Design review of the part built by this model. Coordinates are the model's own, in mm. A direction names the side the tool comes from. Coordinates: 2 decimals unless noted, no trailing zeros. Loops run counter-clockwise (first coordinate to the right, second up) from the corner with the lowest first, then second, coordinate; pieces in that order, holes last.
Q1. Add section C-C on y = -44. Give the boundary of the cut face in (x, z), and give its area (3 significant figures).
Q2. Draft analysis for pull direction Z (two halves, no side actions). For faces 1 (the face through (-0.54, -82.68, -2.44)), 2 (the face through (0, -70, 0)), 3 (the face through (5.15, -53.72, -0.05)), 4 (the face through (-4.76, -46.84, -3.65)), state which applies: released by +Z, released by -Z, zero draft, split by the parting line, or undercut.
Q3. Add section B-B on z = 0. Give the boundary of the cut face in (x, y), and give its area (3 significant figures).
Q4. Machinability: for faces 5 (the face through (5.16, -41.24, -0.05)), 6 (the face through (3, -95, 0)), 7 (the face through (0, -25, 0)), 8 (the face through (-5, -48, 0)), which of the approach directions +Z, -Z, +X, -X, +Y, -Y give a long, thin tool a straight path to every point of the face, cutting with its end or side? Answer none if there is none.
Q5. Wall thickness on probe 1 along Z at (x, y) = (0, -11.25); probe 2 along Y at (x, z) = (-1, 1); probe 3 along Z at (x, y) = (2, -82): over which ranges is each line inside the solid? List them lowest first.
Q6. Add section D-D on y = -16. Give the boundary of the cut face in (x, z), and give its area (3 significant figures).
Q7. For P1, Ø2.5, axis at x = -1, z = 0, coming from the +Y side; P2, Ø1.5, axis at x = 1, z = 0, coming from the -Y side; P3, Ø5, axis at x = 5, y = -25, coming from the +Z side, all flat-tipped, find the tip position at first contact; note any pin that passes through.
Q8. Add section A-A on x = 0. Give the boundary of the cut face in (y, z), and give its area (3 significant figures).
```python
from build123d import *

# Parameters (mm, degrees)
F0_R     = 6
F1_DEPTH = 95
F2_R     = 2.5
F3_DEPTH = 25
F4_R     = 2.5
F5_DEPTH = 25
F7_DEPTH = 12.5


with BuildPart() as f1:
    # F0 (on Front) → F1 (new body)
    with BuildSketch(Plane.XZ):
        Circle(F0_R)
    extrude(amount=F1_DEPTH)

    # F2 (on face) → F3 (cut)
    with BuildSketch(Plane.XZ.offset(95)):
        Circle(F2_R)
    extrude(amount=-F3_DEPTH, mode=Mode.SUBTRACT)

    # F4 (on face) → F5 (cut)
    with BuildSketch(Plane(origin=(0, 0, 0), x_dir=(-1, 0, 0), z_dir=(0, 1, 0))):
        Circle(F4_R)
    extrude(amount=-F5_DEPTH, mode=Mode.SUBTRACT)

    # F6 (on Top) → F7 (cut, symmetric)
    with BuildSketch(Plane.XY):
        with BuildLine():
            Line((11.650951, -37.5), (10, -37.5))
            ThreePointArc((10, -37.5), (6.464466, -38.964466), (5, -42.5))
            Line((5, -42.5), (5, -52.5))
            ThreePointArc((5, -52.5), (6.464466, -56.035534), (10, -57.5))
            Line((10, -57.5), (11.650951, -57.5))
            Line((11.650951, -57.5), (11.650951, -37.5))
        make_face()
        with BuildLine():
            ThreePointArc((-5, -42.5), (-6.464466, -38.964466), (-10, -37.5))
            Line((-10, -37.5), (-11.650951, -37.5))
            Line((-11.650951, -37.5), (-11.650951, -57.5))
            Line((-11.650951, -57.5), (-10, -57.5))
            ThreePointArc((-10, -57.5), (-6.464466, -56.035534), (-5, -52.5))
            Line((-5, -52.5), (-5, -42.5))
        make_face()
    extrude(amount=F7_DEPTH, both=True, mode=Mode.SUBTRACT)


solid = f1.part
```
Entries:
1. outline: (-5, -3.32) arc R6 ccw to (5, -3.32) - (5, 3.32) arc R6 ccw to (-5, 3.32) - close
1. area: 104 mm2
2. face 1: undercut
2. face 2: undercut
2. face 3: zero draft
2. face 4: split by the parting line
3. outline: (-6, -95) - (-2.5, -95) - (-2.5, -70) - (2.5, -70) - (2.5, -95) - (6, -95) - (6, -55.5) arc R5 cw to (5, -52.5) - (5, -42.5) arc R5 cw to (6, -39.5) - (6, 0) - (2.5, 0) - (2.5, -25) - (-2.5, -25) - (-2.5, 0) - (-6, 0) - (-6, -39.5) arc R5 cw to (-5, -42.5) - (-5, -52.5) arc R5 cw to (-6, -55.5) - close
3. area: 862 mm2
4. face 5: +Z, -Z, +X
4. face 6: +Z, -Z, +X, -X, -Y
4. face 7: +Y
4. face 8: +Z, -Z, -X
5. probe 1: z = -6 to -2.5, 2.5 to 6
5. probe 2: y = -70 to -25
5. probe 3: z = -5.66 to -1.5, 1.5 to 5.66
6. outline: circle Ø12 at (0, 0); hole circle Ø5 at (0, 0)
6. area: 93.5 mm2
7. P1: stops at y = -25
7. P2: stops at y = -70
7. P3: stops at z = 5.45
8. outline: (-95, -6) - (0, -6) - (0, -2.5) - (-25, -2.5) - (-25, 2.5) - (0, 2.5) - (0, 6) - (-95, 6) - (-95, 2.5) - (-70, 2.5) - (-70, -2.5) - (-95, -2.5) - close
8. area: 890 mm2
